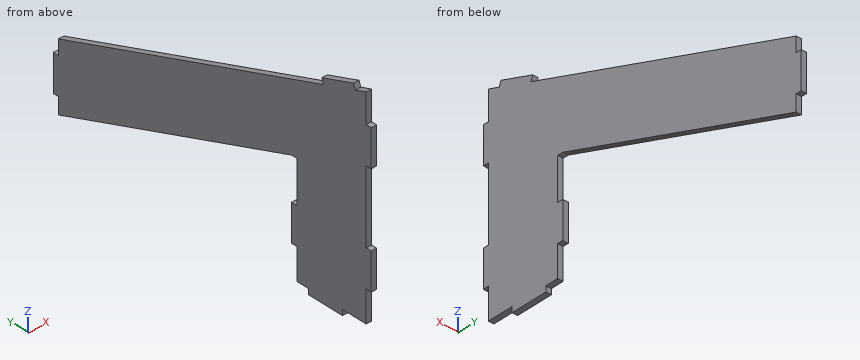
```python
from build123d import *

# Parameters (mm, degrees)
BOSS_EXTRUDE1_DEPTH = 3
CUT_EXTRUDE1_DEPTH  = 267.131484195
SKETCH3_W           = 29.976768642
SKETCH3_H           = 52.268511193
CUT_EXTRUDE2_DEPTH  = 233.651187464
SKETCH5_W           = 11.091910703
SKETCH5_H           = 3
SKETCH5_W_2         = 10
CUT_EXTRUDE4_DEPTH  = 224.001992956
SKETCH6_W           = 20
SKETCH6_H           = 3
CUT_EXTRUDE5_DEPTH  = 224.001992956
SKETCH7_W           = 40
SKETCH7_H           = 3
CUT_EXTRUDE6_DEPTH  = 224.001992956
SKETCH8_W           = 20
SKETCH8_H           = 3
SKETCH8_W_2         = 22.898992834
CUT_EXTRUDE7_DEPTH  = 224.001992956
SKETCH10_W          = 3
SKETCH10_H          = 7
SKETCH10_H_2        = 13.984631039
CUT_EXTRUDE9_DEPTH  = 224.001992956
CUT_EXTRUDE10_REACH = 225.002
SKETCH12_W          = 3
SKETCH12_H          = 20
BOSS_EXTRUDE2_DEPTH = 3


with BuildPart() as part:
    # Sketch1 → Boss-Extrude1 (new body)
    with BuildSketch(Plane(origin=(0, 0, 0), x_dir=(0, 0, -1), z_dir=(1, 0, 0))):
        Polygon((0, 0), (120, 0), (188.404028665, 187.938524157), (68.404028665, 187.938524157), align=None)
    extrude(amount=BOSS_EXTRUDE1_DEPTH)

    # Sketch2 → Cut-Extrude1 (cut, through all)
    with BuildSketch(Plane(origin=(3, 0, 0), x_dir=(0, 0, -1), z_dir=(1, 0, 0))):
        Polygon((188.404028665, 187.938524157), (137.101007166, 46.984631039), (57.101007166, 46.984631039), (108.404028665, 187.938524157), align=None)
    extrude(amount=-CUT_EXTRUDE1_DEPTH, mode=Mode.SUBTRACT)

    # Sketch3 → Cut-Extrude2 (cut, through all)
    with BuildSketch(Plane(origin=(3, 0, 0), x_dir=(0, 0, -1), z_dir=(1, 0, 0))):
        with Locations((134.988384321, 26.134255597)):
            Rectangle(SKETCH3_W, SKETCH3_H)
    extrude(amount=-CUT_EXTRUDE2_DEPTH, mode=Mode.SUBTRACT)

    # Sketch5 → Cut-Extrude4 (cut, through all)
    with BuildSketch(Plane(origin=(3, 0, 0), x_dir=(0, 0, -1), z_dir=(1, 0, 0))):
        with Locations((72.858073314, 186.438524157)):
            Rectangle(SKETCH5_W, SKETCH5_H)
        with Locations((103.404028665, 186.438524157)):
            Rectangle(SKETCH5_W_2, SKETCH5_H)
    extrude(amount=-CUT_EXTRUDE4_DEPTH, mode=Mode.SUBTRACT)

    # Sketch6 → Cut-Extrude5 (cut, through all)
    with BuildSketch(Plane(origin=(3, 0, 0), x_dir=(0, 0, -1), z_dir=(1, 0, 0))):
        with Locations((110, 1.5)):
            Rectangle(SKETCH6_W, SKETCH6_H)
        with Locations((10, 1.5)):
            Rectangle(SKETCH6_W, SKETCH6_H)
    extrude(amount=-CUT_EXTRUDE5_DEPTH, mode=Mode.SUBTRACT)

    # Sketch7 → Cut-Extrude6 (cut, through all)
    with BuildSketch(Plane(origin=(3, 0, 0), x_dir=(0, 0, -1), z_dir=(1, 0, 0))):
        with Locations((60, 1.5)):
            Rectangle(SKETCH7_W, SKETCH7_H)
    extrude(amount=-CUT_EXTRUDE6_DEPTH, mode=Mode.SUBTRACT)

    # Sketch8 → Cut-Extrude7 (cut, through all)
    with BuildSketch(Plane(origin=(3, 0, 0), x_dir=(0, 0, -1), z_dir=(1, 0, 0))):
        with Locations((110, 45.484631039)):
            Rectangle(SKETCH8_W, SKETCH8_H)
        with Locations((68.550503583, 45.484631039)):
            Rectangle(SKETCH8_W_2, SKETCH8_H)
    extrude(amount=-CUT_EXTRUDE7_DEPTH, mode=Mode.SUBTRACT)

    # Sketch10 → Cut-Extrude9 (cut, through all)
    with BuildSketch(Plane(origin=(3, 0, 0), x_dir=(0, 0, -1), z_dir=(1, 0, 0))):
        with Locations((118.5, 40.484631039)):
            Rectangle(SKETCH10_W, SKETCH10_H)
        with Locations((118.5, 9.992315519)):
            Rectangle(SKETCH10_W, SKETCH10_H_2)
    extrude(amount=-CUT_EXTRUDE9_DEPTH, mode=Mode.SUBTRACT)

    # Sketch11 → Cut-Extrude10 (cut, up to next)
    with BuildSketch(Plane.ZY, mode=Mode.PRIVATE) as cut_extrude10_sk1:
        Polygon((-67.312117962, 184.938524157), (-1.091910703, 3), (-4.091910703, 3), (-70.312117962, 184.938524157), align=None)
    cut_extrude10_tool1 = extrude(cut_extrude10_sk1.sketch, amount=-CUT_EXTRUDE10_REACH, mode=Mode.PRIVATE) & part.part
    add(cut_extrude10_tool1.solids().sort_by_distance((0, 93.969262, -35.702014))[0], mode=Mode.SUBTRACT)

    # Sketch12 → Boss-Extrude2 (add)
    with BuildSketch(Plane(origin=(0, -0.964181415, -2.649066665), x_dir=(1, 0, 0), z_dir=(0, 0.34202014332566577, 0.9396926207859095))):
        with Locations((1.5, 21.02606043)):
            Rectangle(SKETCH12_W, SKETCH12_H)
    extrude(amount=BOSS_EXTRUDE2_DEPTH)


solid = part.part
```
Could you check a few things on this model? Use its own coordinates, in mm. Give positions to 0.01 mm unless a question says otherwise; leave off trailing zeros. Loops run counter-clockwise (first coordinate to the right, second up) from the corner with the lowest first, then second, coordinate; pieces in that order, holes last. Notation, with made-up numbers: (30, 0) -> (87, 0) arc R23 ccw to (87, 22) -> close; hole circle Ø10 at (-34.5, 79.5). An arc over 180 degrees is marked (long way). Put each result on its own line as item: value.
(1) Please list where these lines run through material, in increasing order: probe 1 along Y at (x, z) = (1.5, -112); probe 2 along Z at (x, y) = (2.1, 148.5); probe 3 along Z at (x, y) = (1.5, 51). Write a range as [from, to].
Computed:
probe 1: [3, 43.98]
probe 2: [-94.05, -57.05]
probe 3: [-58.56, -21.56]
(2) Imagine slicing it at C-C on y = 99. Write out the boundary of the cut face in (x, z), plus the area to 3 significant figures.
Computed:
outline: (0, -76.03) -> (3, -76.03) -> (3, -39.03) -> (0, -39.03) -> close
area: 111 mm^2
(3) I'm going to push flat-ended pins straight in: pin 1 Ø0.9 at (x, z) = (1.5, -103.5) entering from +Y; pin 2 Ø1 at (x, y) = (1, 54.5) entering from -Z; pin 3 Ø0.9 at (x, y) = (1.5, 1.5) entering from +Z. Where does each tip first touch, or does it pass through?
Computed:
pin 1: y = 184.94
pin 2: z = -60.02
pin 3: z = -20
(4) Imagine slicing it at D-D on z = -104. Write out the boundary of the cut face in (x, y).
Computed:
outline: (0, 3) -> (3, 3) -> (3, 43.98) -> (0, 43.98) -> close; (0, 175.84) -> (3, 175.84) -> (3, 184.94) -> (0, 184.94) -> close
(5) Imagine slicing it at B-B on z = -65. Write out the boundary of the cut face in (x, y), plus the area to 3 significant figures.
Computed:
outline: (0, 3) -> (3, 3) -> (3, 43.98) -> (0, 43.98) -> close; (0, 68.69) -> (3, 68.69) -> (3, 170.34) -> (0, 170.34) -> close
area: 428 mm^2
